Here's how the part is built. I have some questions about the finished solid (model axes, mm). Coordinates: 2 decimals unless noted, no trailing zeros. Write each loop counter-clockwise with the first axis right and the second up, starting at its lowest first coordinate (ties: lowest second). Pieces come first, ordered by that corner, then holes.
Item 1: I'm going to push flat-ended pins straight in: pin 1 Ø1 at (y, z) = (0.5, 59) entering from +X; pin 2 Ø1 at (y, z) = (1, -85) entering from -X. Where does each tip first touch, or does it pass through?
Item 2: If we section it at A-A (z = 113): Please give me the cut outline in (x, y), then the cut area to 3 significant figures.
Item 3: If I drill on line 1 (X direction, y = 1.2, z = 58); line 2 (X direction, y = 0.8, z = 19); line 3 (Z direction, x = -27, y = 0.85), over which ranges is the centre line in solid material (lowest first)?
from build123d import *

# Parameters (mm, degrees)
BOSS_EXTRUDE1_DEPTH = 2


with BuildPart() as part:
    # Sketch1 → Boss-Extrude1 (new body)
    with BuildSketch(Plane(origin=(0, 0, 0), x_dir=(1, 0, 0), z_dir=(0, 1, 0))):
        with BuildLine():
            ThreePointArc((-40.679244353, -103.221523445), (-6.884583356, -132.122739902), (26.910077355, -103.221523111))
            add(Edge.make_bspline(
                [(10.32075615, 135.087420221), (39.402555208, 121.787875107), (48.095792581, 85.931785161), (48.363582245, 1.743673196), (22.570320599, -55.244701587), (26.910077355, -103.221523111)],
                knots=[0, 0, 0, 0, 0.296821126, 0.429544144, 1, 1, 1, 1], degree=3))
            add(Edge.make_bspline(
                [(-10.296198393, 131.704373688), (-7.252650356, 138.974935501), (5.280450445, 141.193491305), (10.32075615, 135.087420221)],
                knots=[0, 0, 0, 0, 1, 1, 1, 1], degree=3))
            add(Edge.make_bspline(
                [(-46.679244317, 103.587421062), (-52.785760987, 121.907427011), (-38.636955581, 157.574381944), (-10.296198393, 131.704373688)],
                knots=[0, 0, 0, 0, 1, 1, 1, 1], degree=3))
            add(Edge.make_bspline(
                [(-40.679244353, -103.221523445), (-48.424660229, -69.464624821), (-5.31250584, -0.275920012), (-54.797034308, 67.469917015), (-46.679244317, 103.587421062)],
                knots=[0, 0, 0, 0, 0.483382248, 1, 1, 1, 1], degree=3))
        make_face()
    extrude(amount=BOSS_EXTRUDE1_DEPTH)


solid = part.part
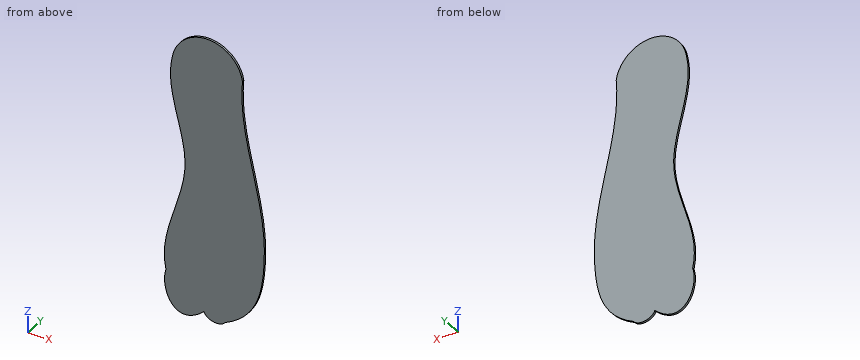
Answer list:
1. pin 1: stops at x = 28.97
1. pin 2: stops at x = -48.2
2. outline: (-37.59, 0) - (23.82, 0) - (23.82, 2) - (-37.59, 2) - close
2. area: 123 mm2
3. line 1: x = -38.38 to 29.05
3. line 2: x = -29.48 to 37.02
3. line 3: z = -140.7 to 125.58
